The model under review builds one solid part; all positions refer to its coordinate system, in mm. A direction names the side the tool comes from. Round coordinates to 2 decimals unless told otherwise and drop trailing zeros. Return JSON: item names as keys, results as strings. Group by question number.
Q1. Draft analysis for pull direction Z (two halves, no side actions). For faces 3 (the face through (0, -16, 0)), 4 (the face through (-5.106, -11.444, -0.67)), 5 (the face through (7, 0, 0)), state which applies: pulls with the +Z half, pulls with the -Z half, needs draft (parallel to the pull), parting line crosses it, or undercut.
Q2. Clearance check with flat-ended pins moving along their axes: pin 1 Ø1.9 at (y, z) = (-8, 5) entering from -X; pin 2 Ø1.5 at (x, z) = (-7, -3.5) entering from +Y; pin 3 Ø1 at (x, z) = (1.5, -2) entering from -Y; pin 4 Ø3 at (y, z) = (-7.5, -5.5) entering from +X. State where each tip first meets the part, or that it passes through.
Q3. To check wall thickness, follow line 1 along X through (y, z) = (-3, -6); line 2 along X through (y, z) = (-3.75, 6.25); line 3 along Y through (x, z) = (3.5, -4). State the ranges of each line that lie inside material, in increasing order.
Q4. For faces 1 (the face through (-7, 0, 0)), 2 (the face through (0, -13, 6)), list the 3-axis set-ups (+Z, -Z, +X, -X, +Y, -Y) from which the entire face can be reached by the end or side of a thin tool; tool diameter is ignored.
from build123d import *

# Parameters (mm, degrees)
F2_W     = 10
F2_H     = 18
F3_DEPTH = 13


with BuildPart() as f1:
    # F0 (on Right) → F1 (revolve)
    with BuildSketch(Plane.YZ):
        with BuildLine():
            Line((-16, 5.15), (0, 5.15))
            Line((0, 5.15), (0, 9))
            add(Edge.make_bspline(
                [(-21, 0), (-21, 5.15), (-16, 8.955878), (0, 9)],
                knots=[0, 0, 0, 0, 22.847319, 22.847319, 22.847319, 22.847319], degree=3))
            Line((-21, 0), (-16, 0))
            Line((-16, 0), (-16, 5.15))
        make_face()
    revolve(axis=Axis((0, -18.5, 0), (0, -1, 0)))

    # F2 (on face) → F3 (cut)
    with BuildSketch(Plane(origin=(0, 0, 0), x_dir=(-1, 0, 0), z_dir=(0, 1, 0))):
        Rectangle(F2_W, F2_H)
    extrude(amount=-F3_DEPTH, mode=Mode.SUBTRACT)


solid = f1.part
Values:
{
 "1": {"face 3": "undercut", "face 4": "undercut", "face 5": "needs draft"},
 "2": {"pin 1": "stops at x = -7.58", "pin 2": "stops at y = 0", "pin 3": "stops at y = -20.71", "pin 4": "stops at x = 7.67"},
 "3": {"line 1": "x = -6.63 to -5, 5 to 6.63", "line 2": "x = -6.35 to -5, 5 to 6.35", "line 3": "y = -18.3 to -13"},
 "4": {"face 1": "+Z, -Z, +X, -X, +Y", "face 2": "+Z, -Z, +Y"}
}
